```python
from build123d import *

# Parameters (mm, degrees)
SKETCH1_W           = 5.162383308
SKETCH1_H           = 20.435052184
BOSS_EXTRUDE1_DEPTH = 1.27
SKETCH2_W           = 0.838933851
SKETCH2_H           = 3.882140463
CUT_EXTRUDE1_DEPTH  = 3.81
SKETCH3_W           = 0.856262928
SKETCH3_H           = 2.429514696
BOSS_EXTRUDE2_DEPTH = 3.81


with BuildPart() as part:
    # Sketch1 → Boss-Extrude1 (new body)
    with BuildSketch(Plane.XY):
        with Locations((-34.98361032, 7.835499756)):
            Rectangle(SKETCH1_W, SKETCH1_H)
    extrude(amount=BOSS_EXTRUDE1_DEPTH)

    # Sketch2 → Cut-Extrude1 (cut)
    with BuildSketch(Plane.ZY.offset(37.564801974)):
        with Locations((0.611191145, 14.932897959)):
            Rectangle(SKETCH2_W, SKETCH2_H)
    extrude(amount=-CUT_EXTRUDE1_DEPTH, mode=Mode.SUBTRACT)

    # Sketch3 → Boss-Extrude2 (add)
    with BuildSketch(Plane(origin=(-32.402418666, 0, 0), x_dir=(0, 0, -1), z_dir=(1, 0, 0))):
        with Locations((-0.669030721, 16.8382685)):
            Rectangle(SKETCH3_W, SKETCH3_H)
    extrude(amount=BOSS_EXTRUDE2_DEPTH)


solid = part.part
```
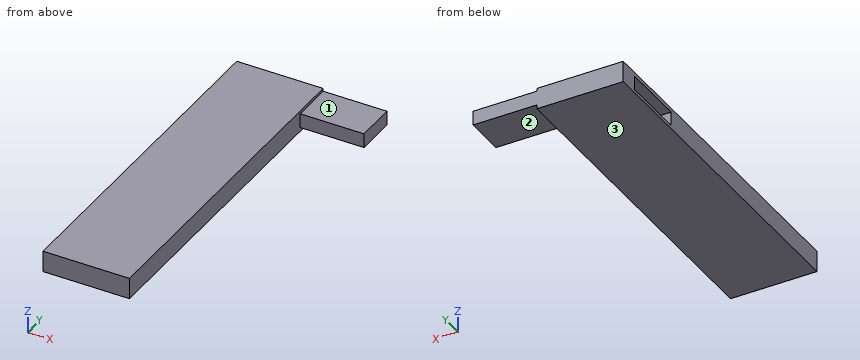
Geometry: final body of the model. Coordinates: model frame, mm. Face numbers are marked on the shaded views. A direction names the side the tool comes from. Round coordinates to 2 decimals unless told otherwise and drop trailing zeros. Loops run counter-clockwise (first coordinate to the right, second up) from the corner with the lowest first, then second, coordinate; pieces in that order, holes last. Notation, with made-up numbers: (25, -25) -> (72, -25) arc R25 ccw to (72, 5) -> close; hole circle Ø11 at (71.25, 69). An arc over 180 degrees is marked (long way). Use one line per item in the form item = value. Start each with the question number.
1) Section A-A on x = -34.75. Output: boundary loops of the cut face in (y, z).
2) Section C-C on y = 9.75. Output: boundary loops of the cut face in (x, z), then the cut area to 3 significant figures.
3) Line query: L1, parallel to Y at x = -36.75, z = 0.3; L2, parallel to X at y = 7.75, z = 0.8; L3, parallel to X at y = 15, z = 0.4. Output: solid intervals per line, ascending.
4) First-contact query: P1, Ø2.5, axis at x = -31, y = 17.5, coming from the -Z side; P2, Ø2.5, axis at x = -30, y = 17, coming from the +Z side. Flat tips, straight axial feed; report the tip coordinate or a pass-through.
5) Access query for the marked faces 1, 2 and 3. Directions: +Z, -Z, +X, -X, +Y, -Y. A direction counts if a zero-diameter tool reaches every point of the face in a straight line with its end or side. Return the directions, or none.
6) Section D-D on x = -29.25. Output: boundary loops of the cut face in (y, z), then the cut area to 3 significant figures.
7) Section B-B on z = 0.8. Output: boundary loops of the cut face in (x, y).
Response:
q1.outline = (-2.38, 0) -> (18.05, 0) -> (18.05, 1.27) -> (-2.38, 1.27) -> close; hole (12.99, 0.19) -> (16.87, 0.19) -> (16.87, 1.03) -> (12.99, 1.03) -> close
q2.outline = (-37.56, 0) -> (-32.4, 0) -> (-32.4, 1.27) -> (-37.56, 1.27) -> close
q2.area = 6.56 mm^2
q3.L1 = -2.38 to 12.99, 16.87 to 18.05
q3.L2 = -37.56 to -32.4
q3.L3 = -33.75 to -32.4
q4.P1 = 0.24
q4.P2 = 1.1
q5.face_1 = +Z, +X, +Y, -Y
q5.face_2 = -Z, +X, +Y, -Y
q5.face_3 = -Z, +X, -X, +Y, -Y
q6.outline = (15.62, 0.24) -> (18.05, 0.24) -> (18.05, 1.1) -> (15.62, 1.1) -> close
q6.area = 2.08 mm^2
q7.outline = (-37.56, -2.38) -> (-32.4, -2.38) -> (-32.4, 15.62) -> (-28.59, 15.62) -> (-28.59, 18.05) -> (-37.56, 18.05) -> (-37.56, 16.87) -> (-33.75, 16.87) -> (-33.75, 12.99) -> (-37.56, 12.99) -> close
